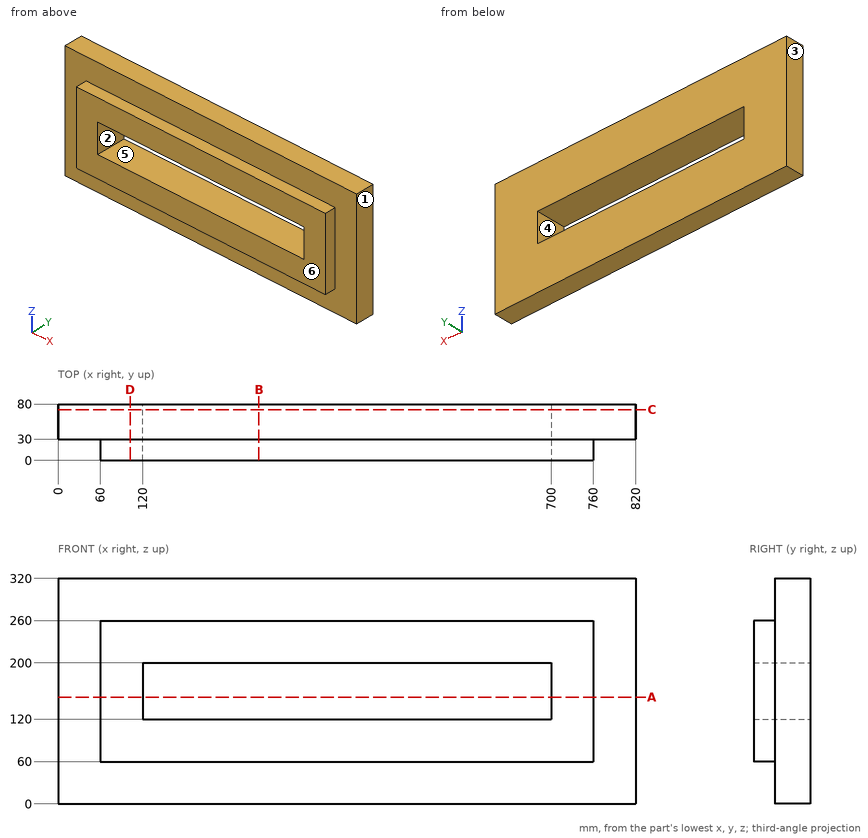
Answer from the drawing. Dimensions are ordinates in mm from the lowest x, y and z of the part. A direction names the side the tool comes from. Round coordinates to 2 decimals unless told otherwise and drop trailing zeros. Write each loop counter-clockwise with the first axis right and the second up, starting at its lowest first coordinate (ties: lowest second). Pieces come first, ordered by that corner, then holes. Notation, with made-up numbers: (79.25, 34.25) -> (98.25, 34.25) arc R3 cw to (98.25, 39.25) -> close; hole circle Ø11 at (63.25, 84.5). An arc over 180 degrees is marked (long way). Answer in a Markdown table with one row per item. Add a question column.
1) Determine the mould class of the marked faces 3, 4, 5 and 6 for opening direction X: pulls with the +X half, pulls with the -X half, needs draft (parallel to the pull), parting line crosses it, or undercut.
2) Which of the six approach directions +Z, -Z, +X, -X, +Y, -Y give full straight-line access (tool end or side, diameter ignored) to the marked faces 1 and 2?
3) Find section D-D, the plane x = 102.5. Determine the outline of the cut face in (y, z), and give its area (3 significant figures).
4) Find section A-A, the plane z = 151.5. Determine the outline of the cut face in (x, y).
5) Given P1, Ø10, axis at y = 24, z = 41, coming from the +X side; P2, Ø15, axis at y = 11.5, z = 172.5, coming from the +X side; P3, Ø6, axis at y = 23, z = 198, coming from the -X side; P4, Ø9, axis at x = 490, y = 7.5, coming from the +Z side, each flat-ended and moving along its own axis, determine where each tip first touches the part or whether it passes through.
6) Find section B-B, the plane x = 285. Determine the outline of the cut face in (y, z), and give its area (3 significant figures).
7) Consider line 1 (Z direction, x = 605.5, y = 23.5); line 2 (X direction, y = 55.5, z = 144.5); line 3 (Z direction, x = 481, y = 31.5). Determine where each line is inside the solid, lowest interval first.
8) Find section C-C, the plane y = 72. Determine the outline of the cut face in (x, z), and give its area (3 significant figures).
Findings below:
| question | item | result |
|---|---|---|
| 1 | face 3 | pulls with the -X half |
| 1 | face 4 | undercut |
| 1 | face 5 | undercut |
| 1 | face 6 | needs draft |
| 2 | face 1 | +Z, -Z, +X, +Y, -Y |
| 2 | face 2 | +Y, -Y |
| 3 | outline | (0, 60) -> (30, 60) -> (30, 0) -> (80, 0) -> (80, 320) -> (30, 320) -> (30, 260) -> (0, 260) -> close |
| 3 | area | 22,000 mm² |
| 4 | outline | (0, 30) -> (60, 30) -> (60, 0) -> (120, 0) -> (120, 80) -> (0, 80) -> close; (700, 0) -> (760, 0) -> (760, 30) -> (820, 30) -> (820, 80) -> (700, 80) -> close |
| 5 | P1 | through |
| 5 | P2 | x = 760 |
| 5 | P3 | x = 60 |
| 5 | P4 | z = 260 |
| 6 | outline | (0, 60) -> (30, 60) -> (30, 0) -> (80, 0) -> (80, 120) -> (0, 120) -> close; (0, 200) -> (80, 200) -> (80, 320) -> (30, 320) -> (30, 260) -> (0, 260) -> close |
| 6 | area | 15,600 mm² |
| 7 | line 1 | 60 to 120, 200 to 260 |
| 7 | line 2 | 0 to 120, 700 to 820 |
| 7 | line 3 | 0 to 120, 200 to 320 |
| 8 | outline | (0, 0) -> (820, 0) -> (820, 320) -> (0, 320) -> close; hole (120, 120) -> (700, 120) -> (700, 200) -> (120, 200) -> close |
| 8 | area | 216,000 mm² |
